Geometry: see drawing. Coordinates: mm, zero at the bounding-box minimum. A direction names the side the tool comes from. Give positions to 0.01 mm unless a question says otherwise; leave off trailing zeros. Write each loop counter-clockwise with the first axis right and the second up, starting at its lowest first coordinate (ties: lowest second). Pieces come first, ordered by that corner, then holes. Notation, with made-up numbers: (17.5, -33) - (21.5, -33) arc R21 ccw to (21.5, -3) - close; hole circle Ø10 at (30, -25.5). An arc over 180 degrees is marked (long way). Use CSV: the item, a comma, the result in double quotes. Start each with the question number.
(1) Draft query along X for the marked faces 3, 4 and 5. Return one class per face: released by +X, released by -X, zero draft, split by the parting line, or undercut.
(2) First-contact query: pin 1 Ø2 at (x, z) = (7, 12.5) entering from +Y; pin 2 Ø8 at (x, y) = (6, 6.5) entering from -Z; pin 3 Ø1.5 at (x, z) = (7, 5.5) entering from +Y. Flat tips, straight axial feed; report the tip coordinate or a pass-through.
(3) Line query: probe 1 along Z at (x, y) = (10, 3.75); probe 2 along Z at (x, y) = (10, 11); probe 3 along X at (y, z) = (14, 13). Output: solid intervals per line, ascending. Write a range as [from, to].
(4) Reachability of the marked faces 1 and 2 from +Z, -Z, +X, -X, +Y, -Y: full face, straight path, thin tool, end or side. Return the list, or none.
(5) Section B-B on y = 7.25. Output: boundary loops of the cut face in (x, z).
(6) Section A-A on z = 8. Output: boundary loops of the cut face in (x, y), and give its area (3 significant figures).
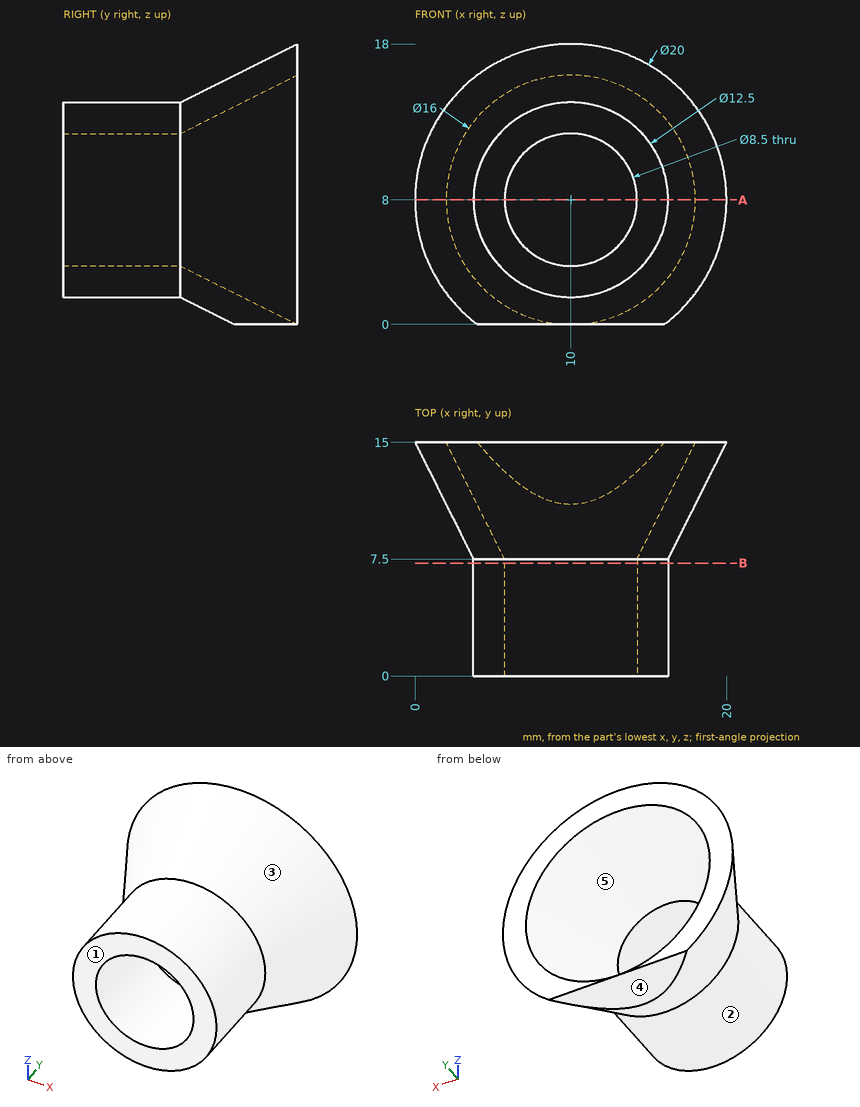
Check values:
1,face 3,"split by the parting line"
1,face 4,"zero draft"
1,face 5,"undercut"
2,pin 1,"stops at y = 11.82"
2,pin 2,"stops at z = 0.79"
2,pin 3,"stops at y = 8.31"
3,probe 1,"z = [1.75, 3.75], [12.25, 14.25]"
3,probe 2,"z = [0, 2], [14, 16]"
3,probe 3,"x = [1.92, 4.41], [15.59, 18.08]"
4,face 1,"+Z, -Z, +X, -X, -Y"
4,face 2,"-Y"
5,outline,"circle Ø12.5 at (10, 8); hole circle Ø8.5 at (10, 8)"
6,outline,"(0, 15) - (3.75, 7.5) - (3.75, 0) - (5.75, 0) - (5.75, 7.5) - (2, 15) - close; (14.25, 0) - (16.25, 0) - (16.25, 7.5) - (20, 15) - (18, 15) - (14.25, 7.5) - close"
6,area,"60.0 mm²"
